from build123d import *

# Parameters (mm, degrees)
SKETCH_1_R      = 34
SKETCH_1_R_2    = 28
EXTRUDE_1_DEPTH = 3.4
EXTRUDE_START   = -7.5
EXTRUDE_2_DEPTH = 7.5


with BuildPart() as part:
    # Эскиз1 → Бобышка-Вытянуть1 (new body)
    with BuildSketch(Plane.XY):
        Circle(SKETCH_1_R)
        Circle(SKETCH_1_R_2, mode=Mode.SUBTRACT)
    extrude(amount=EXTRUDE_1_DEPTH)

    # Эскиз2 → Бобышка-Вытянуть2 (add)
    with BuildSketch(Plane.XY.offset(3.4).offset(EXTRUDE_START)):
        with BuildLine():
            ThreePointArc((-7.5, 26.97684192), (0, 20.8), (7.5, 26.97684192))
            ThreePointArc((7.5, 26.97684192), (0, 28), (-7.5, 26.97684192))
        make_face()
        with BuildLine():
            ThreePointArc((19.612630417, 19.983611489), (18.013328399, 10.4), (27.112630417, 6.993230432))
            ThreePointArc((27.112630417, 6.993230432), (24.248711306, 14), (19.612630417, 19.983611489))
        make_face()
        with BuildLine():
            ThreePointArc((27.112630417, -6.993230432), (18.013328399, -10.4), (19.612630417, -19.983611489))
            ThreePointArc((19.612630417, -19.983611489), (24.248711306, -14), (27.112630417, -6.993230432))
        make_face()
        with BuildLine():
            ThreePointArc((7.5, -26.97684192), (0, -20.8), (-7.5, -26.97684192))
            ThreePointArc((-7.5, -26.97684192), (0, -28), (7.5, -26.97684192))
        make_face()
        with BuildLine():
            ThreePointArc((-19.612630417, -19.983611489), (-18.013328399, -10.4), (-27.112630417, -6.993230432))
            ThreePointArc((-27.112630417, -6.993230432), (-24.248711306, -14), (-19.612630417, -19.983611489))
        make_face()
        with BuildLine():
            ThreePointArc((-27.112630417, 6.993230432), (-18.013328399, 10.4), (-19.612630417, 19.983611489))
            ThreePointArc((-19.612630417, 19.983611489), (-24.248711306, 14), (-27.112630417, 6.993230432))
        make_face()
    extrude(amount=EXTRUDE_2_DEPTH)


solid = part.part
The listing builds one solid part. Answer for the finished solid, in the listing's coordinates (mm). A direction names the side the tool comes from. Coordinates: 2 decimals unless noted, no trailing zeros. Write each loop counter-clockwise with the first axis right and the second up, starting at its lowest first coordinate (ties: lowest second). Pieces come first, ordered by that corner, then holes. Notation, with made-up numbers: (-22, 60) -> (17, 60) arc R35 ccw to (17, 99) -> close; hole circle Ø4 at (31.25, -1). An arc over 180 degrees is marked (long way). One line per question, with ' | ' between items.
1. Section B-B (x = 0) is taken. Determine the outline of the cut face in (y, z), and give its area (3 significant figures).
Verdict:
outline: (-34, 0) -> (-28, 0) -> (-28, -4.1) -> (-20.8, -4.1) -> (-20.8, 3.4) -> (-34, 3.4) -> close; (20.8, -4.1) -> (28, -4.1) -> (28, 0) -> (34, 0) -> (34, 3.4) -> (20.8, 3.4) -> close | area: 149 mm^2
2. For a pull along X with two mould halves and no side action, classify faces 1 (the cylindrical face through (18.28, 28.67, 1.68)), 2 (the flat face through (22, 12, -4.1)), 3 (the cylindrical face through (-0.1, 20.8, -0.4)) as released by +X, released by -X, zero draft, split by the parting line, or undercut.
Verdict:
face 1: split by the parting line | face 2: zero draft | face 3: undercut
3. Given pin 1 Ø5 at (x, y) = (23, 26.5) entering from -Z; pin 2 Ø2 at (x, z) = (24, -2) entering from -Y; pin 3 Ø4 at (y, z) = (5.5, 0.5) entering from +X, each flat-ended and moving along its own axis, determine where each tip first touches the part or whether it passes through.
Verdict:
pin 1: stops at z = 0 | pin 2: stops at y = -15.97 | pin 3: stops at x = 33.82
4. Section C-C (z = 2) is taken. Determine the outline of the cut face in (x, y).
Verdict:
outline: circle Ø68 at (0, 0); hole (-27.11, -6.99) arc R7.64 cw to (-19.61, -19.98) arc R28 ccw to (-7.5, -26.98) arc R7.64 cw to (7.5, -26.98) arc R28 ccw to (19.61, -19.98) arc R7.64 cw to (27.11, -6.99) arc R28 ccw to (27.11, 6.99) arc R7.64 cw to (19.61, 19.98) arc R28 ccw to (7.5, 26.98) arc R7.64 cw to (-7.5, 26.98) arc R28 ccw to (-19.61, 19.98) arc R7.64 cw to (-27.11, 6.99) arc R28 ccw to start
5. Section A-A (y = 0) is taken. Determine the outline of the cut face in (x, z).
Verdict:
outline: (-34, 0) -> (-28, 0) -> (-28, 3.4) -> (-34, 3.4) -> close; (28, 0) -> (34, 0) -> (34, 3.4) -> (28, 3.4) -> close
6. Section D-D (z = -2) is taken. Determine the outline of the cut face in (x, y), and give its area (3 significant figures).
Verdict:
outline: (-27.11, -6.99) arc R28 ccw to (-19.61, -19.98) arc R7.64 ccw to start; (-27.11, 6.99) arc R7.64 ccw to (-19.61, 19.98) arc R28 ccw to start; (-7.5, -26.98) arc R28 ccw to (7.5, -26.98) arc R7.64 ccw to start; (-7.5, 26.98) arc R7.64 ccw to (7.5, 26.98) arc R28 ccw to start; (19.61, -19.98) arc R28 ccw to (27.11, -6.99) arc R7.64 ccw to start; (19.61, 19.98) arc R7.64 ccw to (27.11, 6.99) arc R28 ccw to start | area: 478 mm^2
7. Which of the six approach directions +Z, -Z, +X, -X, +Y, -Y give full straight-line access (tool end or side, diameter ignored) to faces 4 (the cylindrical face through (0, 28, -2)), 5 (the cylindrical face through (-28, 0, 2)), 6 (the cylindrical face through (-24.195, 14.092, -2.079))?
Verdict:
face 4: -Z, +Y | face 5: +Z, -Z | face 6: -Z, -X, +Y
8. Straight lines are drawn through the part: line 1 (X direction, y = -0.5, z = 0.5); line 2 (Z direction, x = -24, y = -15.5); line 3 (Y direction, x = 25.5, z = 0.5). For each, find the intervals that lie inside material, in ascending order.
Verdict:
line 1: x = -34 to -28, 28 to 34 | line 2: z = 0 to 3.4 | line 3: y = -22.49 to -6.63, 6.63 to 22.49
